```python
from build123d import *

# Parameters (mm, degrees)
BOSS_EXTRUDE1_DEPTH = 346.075
SKETCH2_W           = 25.4
SKETCH2_H           = 25.4
BOSS_EXTRUDE2_DEPTH = 76.2


with BuildPart() as part:
    # Sketch1 → Boss-Extrude1 (new body, symmetric)
    with BuildSketch(Plane.XY):
        Polygon((0, 0), (0, 59.055), (-54.864, 59.055), (-54.864, 52.705), (-6.35, 52.705), (-6.35, 0), align=None)
    boss_extrude1 = extrude(amount=BOSS_EXTRUDE1_DEPTH, both=True)

    # Mirror1: Boss-Extrude1 across plane
    add(boss_extrude1.mirror(Plane(origin=(-6.35, 0, 346.075), x_dir=(0, 0, 1), z_dir=(0, 1, 0))))

    # Sketch2 → Boss-Extrude2 (add)
    with BuildSketch(Plane(origin=(0, 0, 0), x_dir=(0, 0, -1), z_dir=(1, 0, 0))):
        with Locations((-257.175, 0)):
            Rectangle(SKETCH2_W, SKETCH2_H)
    boss_extrude2 = extrude(amount=BOSS_EXTRUDE2_DEPTH)

    # Mirror2: Boss-Extrude2 across plane
    add(boss_extrude2.mirror(Plane.XY))


solid = part.part
```
Read the model definition and answer for the solid it produces. Units are mm, in the model's axes. A direction names the side the tool comes from. Round coordinates to 2 decimals unless told otherwise and drop trailing zeros. Loops run counter-clockwise (first coordinate to the right, second up) from the corner with the lowest first, then second, coordinate; pieces in that order, holes last. Notation, with made-up numbers: (-12.5, 23) -> (29.5, 23) arc R18 ccw to (29.5, 52) -> close; hole circle Ø9 at (16.25, -8). An arc over 180 degrees is marked (long way). One line per item, written item: value.
1) Consider L1, parallel to Z at x = 13, y = 6 (3 decimals); L2, parallel to Y at x = -46.5, z = 92.5 (3 decimals); L3, parallel to X at y = -17, z = -158.5. Determine where each line is inside the solid, lowest interval first. Write a range as [from, to].
Answer list:
L1: z = [-269.875, -244.475], [244.475, 269.875]
L2: y = [-59.055, -52.705], [52.705, 59.055]
L3: x = [-6.35, 0]
2) The mould has two halves that part along Y. Classify faces 6 (the face through (-31, 52.705, 5)), 7 (the face through (-5, -9, 346.075)), 8 (the face through (-27, 59.055, 5)), 9 (the face through (38, -12.7, 257)): pulls with the +Y half, pulls with the -Y half, needs draft (parallel to the pull), parting line crosses it, or undercut.
Answer list:
face 6: undercut
face 7: needs draft
face 8: pulls with the +Y half
face 9: pulls with the -Y half
3) Flat-ended cylindrical pins translate along their axes: P1, Ø7.5, axis at x = 22.5, y = 4.5, coming from the -Z side (3 decimals); P2, Ø20.5, axis at x = 37.5, z = 262.5, coming from the +Y side; P3, Ø7.5, axis at x = 41.5, y = -0.5, coming from the +Z side (3 decimals). Find the tip coordinate at first contact, or state that the pin passes through.
Answer list:
P1: stops at z = -269.875
P2: stops at y = 12.7
P3: stops at z = 269.875
4) A cutting plane is placed at D-D (y = -33.5). Determine the outline of the cut face in (x, z) (3 decimals).
Answer list:
outline: (-6.35, -346.075) -> (0, -346.075) -> (0, 346.075) -> (-6.35, 346.075) -> close
5) A cutting plane is placed at A-A (x = 25). Determine the outline of the cut face in (y, z) (3 decimals), and give its area (3 significant figures).
Answer list:
outline: (-12.7, -269.875) -> (12.7, -269.875) -> (12.7, -244.475) -> (-12.7, -244.475) -> close; (-12.7, 244.475) -> (12.7, 244.475) -> (12.7, 269.875) -> (-12.7, 269.875) -> close
area: 1,290 mm²
6) For faces 1 (the face through (38, 0, 269.875)), 2 (the face through (-6.35, -1, 5)), 3 (the face through (38, 0, -269.875)), 4 (the face through (38, 0, -244.475)), 5 (the face through (38, 12.7, 257)), determine the directions among +Z, -Z, +X, -X, +Y, -Y from which every point of the face is accessible in a straight line to the end or side of a thin tool.
Answer list:
face 1: +Z, +X, +Y, -Y
face 2: +Z, -Z, -X
face 3: -Z, +X, +Y, -Y
face 4: +X, +Y, -Y
face 5: +Z, -Z, +X, +Y
7) A cutting plane is placed at B-B (y = -3). Determine the outline of the cut face in (x, z) (3 decimals).
Answer list:
outline: (-6.35, -346.075) -> (0, -346.075) -> (0, -269.875) -> (76.2, -269.875) -> (76.2, -244.475) -> (0, -244.475) -> (0, 244.475) -> (76.2, 244.475) -> (76.2, 269.875) -> (0, 269.875) -> (0, 346.075) -> (-6.35, 346.075) -> close
8) A cutting plane is placed at C-C (z = -204). Determine the outline of the cut face in (x, y) (3 decimals).
Answer list:
outline: (-54.864, -59.055) -> (0, -59.055) -> (0, 59.055) -> (-54.864, 59.055) -> (-54.864, 52.705) -> (-6.35, 52.705) -> (-6.35, -52.705) -> (-54.864, -52.705) -> close
